Part model, mm, in its own coordinate system. Face numbers are marked on the shaded views. Round coordinates to 2 decimals unless told otherwise and drop trailing zeros. Loops run counter-clockwise (first coordinate to the right, second up) from the corner with the lowest first, then second, coordinate; pieces in that order, holes last. Notation, with made-up numbers: M 12.25,50.25 L 17.25,50.25 A38 cw 17.25,89.25 Z; hole C 85.25,-1.75 d9. An arc over 180 degrees is marked long. Put each result on its own line as item: value. Start each with the question number.
1) Slice it at A-A on x = 9. Give the cut face in (y, z).
2) Pull direction Z, two halves, no side cores. Call the marked faces 1, 2 and 3: +Z half, -Z half, draft (parallel to the pull), parting line (faces both ways), or undercut.
3) Slice it at C-C on y = -6. Give the cut face in (x, z), then the cut area to 3 significant figures.
4) Slice it at B-B on z = 33. Give the cut face in (x, y).
5) Probe line 1 along Z through (x, y) = (9, -2.25); line 2 along Z through (x, y) = (35.5, -5); line 3 along X through (y, z) = (-2.5, 39). List the from-to ranges inside material, lowest first.
6) Drop a flat-ended pin along its axis: pin 1 Ø3 at (x, z) = (9, 33) entering from +Y. Give the stop position or say it passes through.
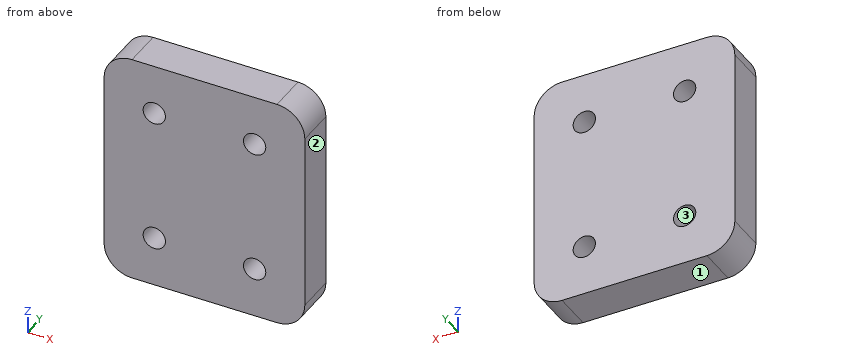
```python
from build123d import *

# Parameters (mm, degrees)
F0_W     = 36
F0_H     = 42
F0_R     = 2
F1_DEPTH = 7
F2_R     = 5


with BuildPart() as f1:
    # F0 (on Front) → F1 (new body)
    with BuildSketch(Plane.XZ):
        with Locations((18, 21)):
            Rectangle(F0_W, F0_H)
        with Locations((9, 9)):
            Circle(F0_R, mode=Mode.SUBTRACT)
        with Locations((27, 9)):
            Circle(F0_R, mode=Mode.SUBTRACT)
        with Locations((9, 33)):
            Circle(F0_R, mode=Mode.SUBTRACT)
        with Locations((27, 33)):
            Circle(F0_R, mode=Mode.SUBTRACT)
    extrude(amount=F1_DEPTH)

    # F2
    f2_edges = [f1.edges().sort_by_distance(p)[0] for p in [
        (0, -3.5, 42),
        (0, -3.5, 0),
        (36, -3.5, 0),
        (36, -3.5, 42),
    ]]
    fillet(f2_edges, radius=F2_R)


solid = f1.part
```
Recorded:
1. outline: M -7,0 L 0,0 L 0,7 L -7,7 Z; M -7,11 L 0,11 L 0,31 L -7,31 Z; M -7,35 L 0,35 L 0,42 L -7,42 Z
2. face 1: -Z half
2. face 2: draft
2. face 3: undercut
3. outline: M 0,5 A5 ccw 5,0 L 31,0 A5 ccw 36,5 L 36,37 A5 ccw 31,42 L 5,42 A5 ccw 0,37 Z; hole C 9,9 d4; hole C 9,33 d4; hole C 27,9 d4; hole C 27,33 d4
3. area: 1,440 mm2
4. outline: M 0,-7 L 7,-7 L 7,0 L 0,0 Z; M 11,-7 L 25,-7 L 25,0 L 11,0 Z; M 29,-7 L 36,-7 L 36,0 L 29,0 Z
5. line 1: z = 0 to 7, 11 to 31, 35 to 42
5. line 2: z = 2.82 to 39.18
5. line 3: x = 0.42 to 35.58
6. pin 1: passes through
